from build123d import *

# Parameters (mm, degrees)
EXTRUDE_THIN1_DEPTH      = 60
EXTRUDE_THIN1_DEPTH_BACK = 60
SKETCH1_W                = 25
SKETCH1_H                = 25
SKETCH1_W_2              = 21
SKETCH1_H_2              = 21
FILLET1_R                = 2
SKETCH2_R                = 4
CUT_EXTRUDE1_DEPTH       = 67.191011474


with BuildPart() as part:
    # Sketch1 → Extrude-Thin1 (new, two sides: drawn at the far end of the back side and taken through both)
    with BuildSketch(Plane.XY.offset(-EXTRUDE_THIN1_DEPTH_BACK)):
        Rectangle(SKETCH1_W, SKETCH1_H)
        Rectangle(SKETCH1_W_2, SKETCH1_H_2, mode=Mode.SUBTRACT)
    extrude(amount=EXTRUDE_THIN1_DEPTH + EXTRUDE_THIN1_DEPTH_BACK)

    # Fillet1
    fillet1_edges = [part.edges().sort_by_distance(p)[0] for p in [
        (12.5, -12.5, 0),
        (-12.5, -12.5, 0),
        (-12.5, 12.5, 0),
        (12.5, 12.5, 0),
    ]]
    fillet(fillet1_edges, radius=FILLET1_R)

    # Sketch2 → Cut-Extrude1 (cut, through all)
    with BuildSketch(Plane(origin=(12.5, 0, 0), x_dir=(0, 0, -1), z_dir=(1, 0, 0))):
        with Locations((-45, 0)):
            Circle(SKETCH2_R)
        with Locations((45, 0)):
            Circle(SKETCH2_R)
    extrude(amount=-CUT_EXTRUDE1_DEPTH, mode=Mode.SUBTRACT)


solid = part.part
Work out the finished part from the listing and answer in its coordinate system (mm). A direction names the side the tool comes from. Give positions to 0.01 mm unless a question says otherwise; leave off trailing zeros. Write each loop counter-clockwise with the first axis right and the second up, starting at its lowest first coordinate (ties: lowest second). Pieces come first, ordered by that corner, then holes. Notation, with made-up numbers: (75.25, 3.25) - (122.25, 3.25) arc R25 cw to (122.25, 30.25) - close; hole circle Ø2 at (37, -36.75). An arc over 180 degrees is marked (long way). One line per item, written item: value. Start each with the question number.
1. For faces 4 (the cylindrical face through (-11.93, -11.9, 0.84)), 5 (the flat face through (-10.5, 0, -1)), determine the directions among +Z, -Z, +X, -X, +Y, -Y from which every point of the face is accessible in a straight line to the end or side of a thin tool.
2. Find section B-B (y = 0). Write down the section's boundary in (x, z).
3. Find section A-A (x = 4.75). Write down the section's boundary in (y, z), then the cut area to 3 significant figures.
4. For a pull along Y with two mould halves and no side action, classify faces 1 (the flat face through (0, -10.5, -1)), 2 (the flat face through (0, -12.5, -1)), 3 (the flat face through (12.5, 0, -1)) as +Y half, -Y half, draft (parallel to the pull), parting line (faces both ways), or undercut.
5. Given pin 1 (13 mm diameter, centred on y = 0, z = 45, fed in from -X); pin 2 (2 mm diameter, centred on x = 2.5, y = 8, fed in from +Z), each flat-ended and moving along its own axis, determine where each tip first touches the part or whether it passes through.
6. Consider probe 1 along X at (y, z) = (1.5, 18.5); probe 2 along Y at (x, z) = (-11.6, -45). Determine where each line is inside the solid, lowest interval first.
7. Find section C-C (z = -45). Write down the section's boundary in (x, y), then the cut area to 3 significant figures.
Geometry results:
1. face 4: +Z, -Z, -X, -Y
1. face 5: +Z, -Z
2. outline: (-12.5, -60) - (-10.5, -60) - (-10.5, -49) - (-12.5, -49) - close; (-12.5, -41) - (-10.5, -41) - (-10.5, 41) - (-12.5, 41) - close; (-12.5, 49) - (-10.5, 49) - (-10.5, 60) - (-12.5, 60) - close; (10.5, -60) - (12.5, -60) - (12.5, -49) - (10.5, -49) - close; (10.5, -41) - (12.5, -41) - (12.5, 41) - (10.5, 41) - close; (10.5, 49) - (12.5, 49) - (12.5, 60) - (10.5, 60) - close
3. outline: (-12.5, -60) - (-10.5, -60) - (-10.5, 60) - (-12.5, 60) - close; (10.5, -60) - (12.5, -60) - (12.5, 60) - (10.5, 60) - close
3. area: 480 mm2
4. face 1: undercut
4. face 2: -Y half
4. face 3: draft
5. pin 1: x = -12.5
5. pin 2: through
6. probe 1: -12.5 to -10.5, 10.5 to 12.5
6. probe 2: -12.17 to -4, 4 to 12.17
7. outline: (-12.5, -10.5) arc R2 ccw to (-10.5, -12.5) - (10.5, -12.5) arc R2 ccw to (12.5, -10.5) - (12.5, -4) - (10.5, -4) - (10.5, -10.5) - (-10.5, -10.5) - (-10.5, -4) - (-12.5, -4) - close; (-12.5, 4) - (-10.5, 4) - (-10.5, 10.5) - (10.5, 10.5) - (10.5, 4) - (12.5, 4) - (12.5, 10.5) arc R2 ccw to (10.5, 12.5) - (-10.5, 12.5) arc R2 ccw to (-12.5, 10.5) - close
7. area: 149 mm2
